The figure shows three views and two pictorial views of one solid part (mm, origin at its lowest corner). Answer the questions. A direction names the side the tool comes from. Give positions to 0.01 mm unless a question says otherwise; leave off trailing zeros. Order: outer loops, then holes, each group sorted by start corner. A loop starts at its lowest first (then second) coordinate and runs counter-clockwise, first axis right, second up. Notation, with made-up numbers: (-30, -0.5) -> (26, -0.5) arc R22 ccw to (26, 33.5) -> close; hole circle Ø6 at (-39, 24.25). An arc over 180 degrees is marked (long way). One line per item, written item: value. Start each with the question number.
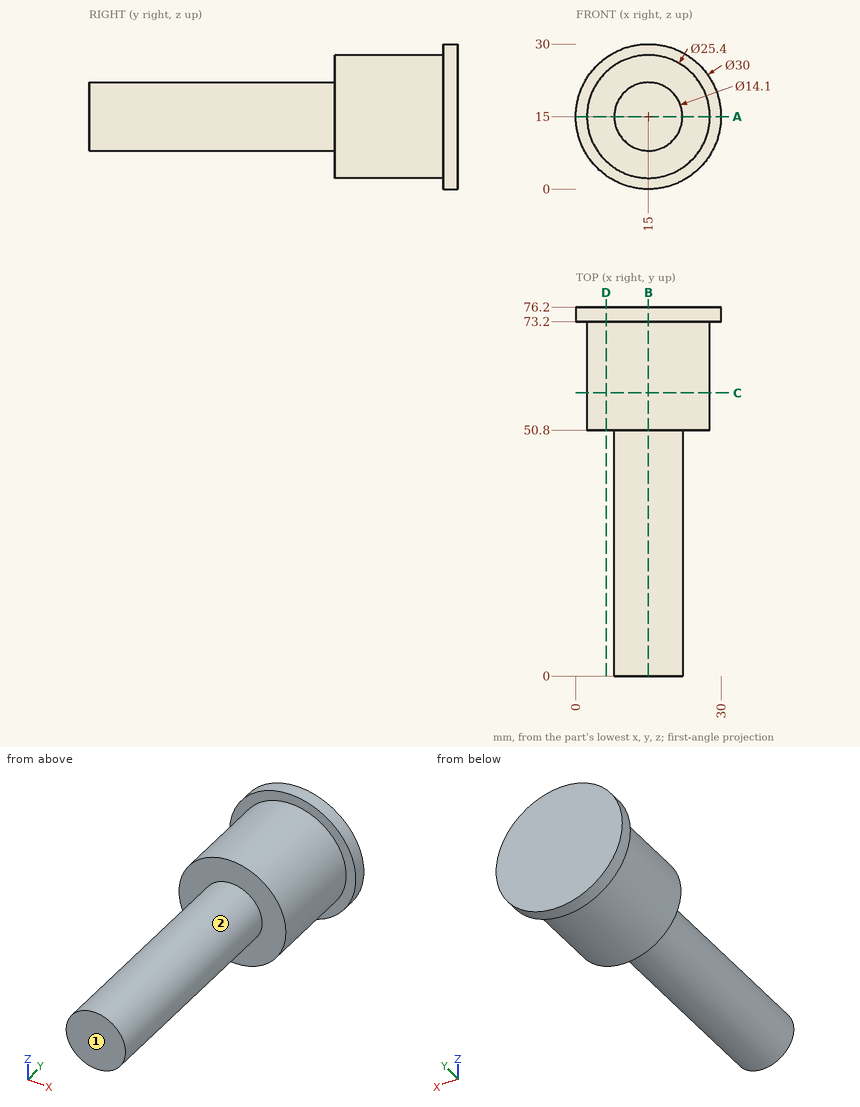
Item 1: Find section A-A on z = 15. Write down the section's boundary in (x, y).
Item 2: Find section B-B on x = 15. Write down the section's boundary in (y, z), then the cut area to 3 significant figures.
Item 3: Flat-ended cylindrical pins translate along their axes: pin 1 (1 mm diameter, centred on x = 9.5, z = 5.5, fed in from -Y); pin 2 (8 mm diameter, centred on y = 68, z = 16, fed in from +X); pin 3 (4 mm diameter, centred on y = 62.5, z = 12.5, fed in from -X). Find the tip coordinate at first contact, or state that the pin passes through.
Item 4: Find the intervals of material crossed by line 1 (Y direction, x = 4.5, z = 18); line 2 (Z direction, x = 15.5, y = 72); line 3 (Y direction, x = 26, z = 8), in increasing order. Write a range as from..to.
Item 5: Find section C-C on y = 58.5. Write down the section's boundary in (x, z), then the cut area to 3 significant figures.
Item 6: A tool of negligible diameter and unlimited length cuts with its end or side. For the marked faces 1 and 2, from which of +Z, -Z, +X, -X, +Y, -Y can it reach the whole face along a straight path? Write none if from no direction.
Item 7: Find section D-D on x = 6.25. Write down the section's boundary in (y, z), then the cut area to 3 significant figures.
Checks:
1. outline: (0, 73.2) -> (2.3, 73.2) -> (2.3, 50.8) -> (7.95, 50.8) -> (7.95, 0) -> (22.05, 0) -> (22.05, 50.8) -> (27.7, 50.8) -> (27.7, 73.2) -> (30, 73.2) -> (30, 76.2) -> (0, 76.2) -> close
2. outline: (0, 7.95) -> (50.8, 7.95) -> (50.8, 2.3) -> (73.2, 2.3) -> (73.2, 0) -> (76.2, 0) -> (76.2, 30) -> (73.2, 30) -> (73.2, 27.7) -> (50.8, 27.7) -> (50.8, 22.05) -> (0, 22.05) -> close
2. area: 1,380 mm2
3. pin 1: y = 50.8
3. pin 2: x = 27.7
3. pin 3: x = 2.31
4. line 1: 50.8..76.2
4. line 2: 2.31..27.69
4. line 3: 73.2..76.2
5. outline: circle Ø25.4 at (15, 15)
5. area: 507 mm2
6. face 1: +Z, -Z, +X, -X, -Y
6. face 2: -Y
7. outline: (50.8, 5.8) -> (73.2, 5.8) -> (73.2, 2.82) -> (76.2, 2.82) -> (76.2, 27.18) -> (73.2, 27.18) -> (73.2, 24.2) -> (50.8, 24.2) -> close
7. area: 485 mm2
